from build123d import *

# Parameters (mm, degrees)
BOSS_EXTRUDE1_DEPTH                            = 60
CSK_FOR_M3_FLAT_HEAD_MACHINE_SCREW1_AT_2_COUNT = 2
CSK_FOR_M3_FLAT_HEAD_MACHINE_SCREW1_AT_2_PITCH = 20
CSK_FOR_M3_FLAT_HEAD_MACHINE_SCREW1_AT_3_COUNT = 2
CSK_FOR_M3_FLAT_HEAD_MACHINE_SCREW1_AT_3_PITCH = 28.284271247
CSK_FOR_M3_FLAT_HEAD_MACHINE_SCREW1_AT_4_COUNT = 2
CSK_FOR_M3_FLAT_HEAD_MACHINE_SCREW1_AT_4_PITCH = 20
M5_CLEARANCE_HOLE1_AT_2_COUNT                  = 2
M5_CLEARANCE_HOLE1_AT_2_PITCH                  = 20
M5_CLEARANCE_HOLE1_AT_3_COUNT                  = 2
M5_CLEARANCE_HOLE1_AT_3_PITCH                  = 40


with BuildPart() as part:
    # Sketch1 → Boss-Extrude1 (new body)
    with BuildSketch(Plane.XY):
        with BuildLine():
            Line((-21.945528184, 16.707726181), (-21.945528184, -18.792273819))
            ThreePointArc((-21.945528184, -18.792273819), (-21.652634965, -19.4993806), (-20.945528184, -19.792273819))
            Line((-20.945528184, -19.792273819), (14.554471816, -19.792273819))
            Line((14.554471816, -19.792273819), (15.054471816, -19.292273819))
            Line((15.054471816, -19.292273819), (15.054471816, -15.292273819))
            Line((15.054471816, -15.292273819), (14.554471816, -14.792273819))
            Line((14.554471816, -14.792273819), (-14.445528184, -14.792273819))
            ThreePointArc((-14.445528184, -14.792273819), (-16.213295137, -14.060040772), (-16.945528184, -12.292273819))
            Line((-16.945528184, -12.292273819), (-16.945528184, 16.707726181))
            Line((-16.945528184, 16.707726181), (-17.445528184, 17.207726181))
            Line((-17.445528184, 17.207726181), (-21.445528184, 17.207726181))
            Line((-21.445528184, 17.207726181), (-21.945528184, 16.707726181))
        make_face()
    extrude(amount=BOSS_EXTRUDE1_DEPTH)

    # Sketch3 → CSK for M3 Flat Head Machine Screw1 (revolve, cut)
    with BuildSketch(Plane(origin=(-11.295528184, -14.792273819, 40), x_dir=(0, 0, 1), z_dir=(1, 0, 0))):
        Polygon((0, 0), (0, 5), (2, 5), (1.7, 4.7), (1.7, 1.95), (3.65, 0), align=None)
    csk_for_m3_flat_head_machine_screw1 = revolve(axis=Axis((-11.295528184, -8.442273819, 40), (0, -1, 0)), mode=Mode.SUBTRACT)

    # CSK for M3 Flat Head Machine Screw1 at 2: CSK for M3 Flat Head Machine Screw1 ×2
    with Locations(*[(i * CSK_FOR_M3_FLAT_HEAD_MACHINE_SCREW1_AT_2_PITCH, 0, 0) for i in range(1, CSK_FOR_M3_FLAT_HEAD_MACHINE_SCREW1_AT_2_COUNT)]):
        add(csk_for_m3_flat_head_machine_screw1, mode=Mode.SUBTRACT)

    # CSK for M3 Flat Head Machine Screw1 at 3: CSK for M3 Flat Head Machine Screw1 ×2
    with Locations(*[Vector(0.7071067811865475, 0, -0.7071067811865476) * (i * CSK_FOR_M3_FLAT_HEAD_MACHINE_SCREW1_AT_3_PITCH) for i in range(1, CSK_FOR_M3_FLAT_HEAD_MACHINE_SCREW1_AT_3_COUNT)]):
        add(csk_for_m3_flat_head_machine_screw1, mode=Mode.SUBTRACT)

    # CSK for M3 Flat Head Machine Screw1 at 4: CSK for M3 Flat Head Machine Screw1 ×2
    with Locations(*[(0, 0, -i * CSK_FOR_M3_FLAT_HEAD_MACHINE_SCREW1_AT_4_PITCH) for i in range(1, CSK_FOR_M3_FLAT_HEAD_MACHINE_SCREW1_AT_4_COUNT)]):
        add(csk_for_m3_flat_head_machine_screw1, mode=Mode.SUBTRACT)

    # Sketch5 → M5 Clearance Hole1 (revolve, cut)
    with BuildSketch(Plane(origin=(-16.945528184, 7.207726181, 50), x_dir=(0, 0, -1), z_dir=(0, 1, 0))):
        Polygon((0, 0), (0, 5), (3.125, 5), (2.75, 4.625), (2.75, 0.375), (3.125, 0), align=None)
    m5_clearance_hole1 = revolve(axis=Axis((-10.595528184, 7.207726181, 50), (-1, 0, 0)), mode=Mode.SUBTRACT)

    # M5 Clearance Hole1 at 2: M5 Clearance Hole1 ×2
    with Locations(*[(0, 0, -i * M5_CLEARANCE_HOLE1_AT_2_PITCH) for i in range(1, M5_CLEARANCE_HOLE1_AT_2_COUNT)]):
        add(m5_clearance_hole1, mode=Mode.SUBTRACT)

    # M5 Clearance Hole1 at 3: M5 Clearance Hole1 ×2
    with Locations(*[(0, 0, -i * M5_CLEARANCE_HOLE1_AT_3_PITCH) for i in range(1, M5_CLEARANCE_HOLE1_AT_3_COUNT)]):
        add(m5_clearance_hole1, mode=Mode.SUBTRACT)


solid = part.part
Design review of the part built by this model. Coordinates are the model's own, in mm. A direction names the side the tool comes from. Round coordinates to 2 decimals unless told otherwise and drop trailing zeros. Write each loop counter-clockwise with the first axis right and the second up, starting at its lowest first coordinate (ties: lowest second). Pieces come first, ordered by that corner, then holes. Notation, with made-up numbers: (44.5, 26) -> (72.5, 26) arc R27 cw to (72.5, 61) -> close; hole circle Ø4 at (-6.75, 17). An arc over 180 degrees is marked (long way). One line per item, written item: value. Start each with the question number.
Q1. Tool access review of faces 1 (the face through (-19.416, 9.647, 8.731)), 2 (the face through (-16.946, 2, 30)): name each direction out of +Z, -Z, +X, -X, +Y, -Y from which nothing blocks a thin tool from reaching the whole face with its end or side.
Q2. Add section B-B (z = 40). Give the boundary of the cut face in (x, y), then the cut area to 3 significant figures.
Q3. Add section D-D (y = 8). State how many separate pieces and enclosed holes the cut face has, then the cut area to 3 significant figures.
Q4. Insertion check: P1, Ø6, axis at y = -6, z = 18.5, coming from the +X side; P2, Ø14.5, axis at x = -5.5, z = 43.5, coming from the +Y side; P3, Ø2.5, axis at x = 8.7, z = 40, coming from the +Y side; P4, Ø4, axis at x = -11.3, z = 20, coming from the +Y side. Each pin has a flat end and moves straight along its axis. Give the tip position at first contact, or say it passes through.
Q5. Add section C-C (z = 55). Give the boundary of the cut face in (x, y), then the cut area to 3 significant figures.
Q6. The part is to be moulded in two halves that separate along X. For faces 3 (the face through (-16.194, -14.079, 29.58)), 4 (the face through (8.63, -18.1, 18.3)), 5 (the face through (-3, -19.792, 30)), 6 (the face through (-10.598, -16.62, 41.683)), say which applies: pulls with the +X half, pulls with the -X half, needs draft (parallel to the pull), parting line crosses it, or undercut.
Q7. To check wall thickness, follow probe 1 along X at (y, z) = (-17, 20); probe 2 along Z at (x, y) = (-17, 8.5); probe 3 along X at (y, z) = (3, 6). State the ranges of each line that lie inside material, in increasing order.
Q8. Add section A-A (z = 30). Give the boundary of the cut face in (x, y), then the cut area to 3 significant figures.
Response:
1. face 1: +X, -X
1. face 2: +Z, -Z, +X, +Y
2. outline: (-21.95, -18.79) arc R1 ccw to (-20.95, -19.79) -> (-13.3, -19.79) -> (-13, -19.49) -> (-13, -16.74) -> (-14.95, -14.79) -> (-14.45, -14.79) arc R2.5 cw to (-16.95, -12.29) -> (-16.95, 16.71) -> (-17.45, 17.21) -> (-21.45, 17.21) -> (-21.95, 16.71) -> close; (-9.6, -19.49) -> (-9.3, -19.79) -> (6.7, -19.79) -> (7, -19.49) -> (7, -16.74) -> (5.05, -14.79) -> (-7.65, -14.79) -> (-9.6, -16.74) -> close; (10.4, -19.49) -> (10.7, -19.79) -> (14.55, -19.79) -> (15.05, -19.29) -> (15.05, -15.29) -> (14.55, -14.79) -> (12.35, -14.79) -> (10.4, -16.74) -> close
2. area: 304 mm^2
3. separate pieces: 4
3. enclosed holes: 0
3. area: 220 mm^2
4. P1: stops at x = -16.95
4. P2: stops at y = -14.79
4. P3: passes through
4. P4: stops at y = -16.44
5. outline: (-21.95, -18.79) arc R1 ccw to (-20.95, -19.79) -> (14.55, -19.79) -> (15.05, -19.29) -> (15.05, -15.29) -> (14.55, -14.79) -> (-14.45, -14.79) arc R2.5 cw to (-16.95, -12.29) -> (-16.95, 16.71) -> (-17.45, 17.21) -> (-21.45, 17.21) -> (-21.95, 16.71) -> close
5. area: 346 mm^2
6. face 3: pulls with the +X half
6. face 4: undercut
6. face 5: needs draft
6. face 6: undercut
7. probe 1: x = -21.95 to -13, -9.6 to 7, 10.4 to 15.05
7. probe 2: z = 0 to 7.21, 12.79 to 27.21, 32.79 to 47.21, 52.79 to 60
7. probe 3: x = -21.95 to -16.95
8. outline: (-21.95, -18.79) arc R1 ccw to (-20.95, -19.79) -> (14.55, -19.79) -> (15.05, -19.29) -> (15.05, -15.29) -> (14.55, -14.79) -> (-14.45, -14.79) arc R2.5 cw to (-16.95, -12.29) -> (-16.95, 4.08) -> (-17.32, 4.46) -> (-21.57, 4.46) -> (-21.95, 4.08) -> close; (-21.95, 10.33) -> (-21.57, 9.96) -> (-17.32, 9.96) -> (-16.95, 10.33) -> (-16.95, 16.71) -> (-17.45, 17.21) -> (-21.45, 17.21) -> (-21.95, 16.71) -> close
8. area: 318 mm^2
